Geometry: final body of the model. Coordinates: model frame, mm. A direction names the side the tool comes from. Coordinates: 2 decimals unless noted, no trailing zeros. Order: outer loops, then holes, each group sorted by start corner. A loop starts at its lowest first (then second) coordinate and runs counter-clockwise, first axis right, second up. Notation, with made-up numbers: (82.5, 54.25) -> (87.5, 54.25) arc R29 cw to (87.5, 82.25) -> close; hole circle Ø4 at (62.25, 61). An arc over 180 degrees is marked (long way). Use one line per item in the form item = value.
```python
from build123d import *

# Parameters (mm, degrees)
SKETCH1_W           = 12
SKETCH1_H           = 17
BOSS_EXTRUDE1_DEPTH = 13
SKETCH2_W           = 15
SKETCH2_H           = 21
BOSS_EXTRUDE2_DEPTH = 2
FILLET1_R           = 1


with BuildPart() as part:
    # Sketch1 → Boss-Extrude1 (new body)
    with BuildSketch(Plane.XY):
        Rectangle(SKETCH1_W, SKETCH1_H)
    extrude(amount=BOSS_EXTRUDE1_DEPTH)

    # Sketch2 → Boss-Extrude2 (add)
    with BuildSketch(Plane.XY):
        Rectangle(SKETCH2_W, SKETCH2_H)
    extrude(amount=BOSS_EXTRUDE2_DEPTH)

    # Fillet1
    fillet1_edges = [part.edges().sort_by_distance(p)[0] for p in [
        (-7.5, 10.5, 1),
        (-7.5, -10.5, 1),
        (7.5, -10.5, 1),
        (7.5, 10.5, 1),
    ]]
    fillet(fillet1_edges, radius=FILLET1_R)


solid = part.part
```
1) Access query for faces 1 (the flat face through (-6, 0, 7)), 2 (the flat face through (0, 0, 13)), 3 (the flat face through (0, -8.5, 7)), 4 (the flat face through (0, 8.5, 7)), 5 (the flat face through (6, 0, 7)). Directions: +Z, -Z, +X, -X, +Y, -Y. A direction counts if a zero-diameter tool reaches every point of the face in a straight line with its end or side. Return the directions, or none.
Results found:
face_1 = +Z, -X, +Y, -Y
face_2 = +Z, +X, -X, +Y, -Y
face_3 = +Z, +X, -X, -Y
face_4 = +Z, +X, -X, +Y
face_5 = +Z, +X, +Y, -Y
2) Section C-C, the plane z = 2.5. Output: boundary loops of the cut face in (x, y), and give its area (3 significant figures).
Results found:
outline = (-6, -8.5) -> (6, -8.5) -> (6, 8.5) -> (-6, 8.5) -> close
area = 204 mm2
3) Contact query for flat-ended pins moving along their axis: P1, Ø5.5, axis at y = -1.5, z = 9.5, coming from the +X side; P2, Ø1, axis at y = 4.5, z = 5, coming from the -X side; P3, Ø6, axis at x = 3, z = 3, coming from the -Y side. Output: stop coordinate, or through.
Results found:
P1 = 6
P2 = -6
P3 = -10.5
4) Section A-A, the plane x = 2.5. Output: boundary loops of the cut face in (y, z), and give its area (3 significant figures).
Results found:
outline = (-10.5, 0) -> (10.5, 0) -> (10.5, 2) -> (8.5, 2) -> (8.5, 13) -> (-8.5, 13) -> (-8.5, 2) -> (-10.5, 2) -> close
area = 229 mm2
5) Material intervals for probe 1 along Y at (x, z) = (1.75, 2.5); probe 2 along X at (y, z) = (-6.5, 9.5); probe 3 along Z at (x, y) = (6, 9), sorted ascending. Write a range as from..to.
Results found:
probe_1 = -8.5..8.5
probe_2 = -6..6
probe_3 = 0..2
6) Section B-B, the plane y = 6. Output: boundary loops of the cut face in (x, z).
Results found:
outline = (-7.5, 0) -> (7.5, 0) -> (7.5, 2) -> (6, 2) -> (6, 13) -> (-6, 13) -> (-6, 2) -> (-7.5, 2) -> close
